Model file for the job. Use its own axes, mm. A direction names the side the tool comes from. Give positions to 0.01 mm unless a question says otherwise; leave off trailing zeros. Loops run counter-clockwise (first coordinate to the right, second up) from the corner with the lowest first, then second, coordinate; pieces in that order, holes last. Notation, with made-up numbers: M -22.75,-20.5 L 16.25,-20.5 A29 ccw 16.25,10.5 Z; hole C -24,-7.75 d8. An arc over 180 degrees is marked long. Answer in a Markdown table with one row per item.
```python
from build123d import *

# Parameters (mm, degrees)
CUT_EXTRUDE1_DEPTH = 1


with BuildPart() as part:
    # Sketch1 → Revolve1 (revolve)
    with BuildSketch(Plane(origin=(0, 0, 0), x_dir=(0, 0, -1), z_dir=(1, 0, 0)), mode=Mode.PRIVATE) as revolve1_sk:
        Polygon((0, 2.5), (0, 4.5), (-0.5, 5), (-1.5, 5), (-1.5, 4), (-12.4, 4), (-12.9, 3.5), (-12.9, 1), (-8, 1), (-8, 2.5), align=None)
    revolve(revolve1_sk.sketch.rotate(Axis((0, 0, 0), (0, 0, -1)), 90), axis=Axis((0, 0, 0), (0, 0, -1)))

    # Sketch2 → Cut-Extrude1 (cut)
    with BuildSketch(Plane(origin=(0, 4, 0), x_dir=(1, 0, 0), z_dir=(0, 1, 0))):
        with BuildLine():
            Line((-1, -12.9), (-1, -4.5))
            ThreePointArc((-1, -4.5), (0, -3.5), (1, -4.5))
            Line((1, -4.5), (1, -12.9))
            ThreePointArc((1, -12.9), (0, -13.9), (-1, -12.9))
        make_face()
    extrude(amount=-CUT_EXTRUDE1_DEPTH, mode=Mode.SUBTRACT)


solid = part.part
```
Q1. 3-axis set-ups, long thin cutter, end or side, ignore diameter. For faces 1 (the face through (-2.5, -0.1, 3.9)), 2 (the face through (2.15, -3.373, 7.026)), 3 (the face through (-1, 3.4, 8.8)), 4 (the face through (-2, 2, 0)): which of +Z, -Z, +X, -X, +Y, -Y reach the whole face in a straight line?
Reported:
| item | result |
|---|---|
| face 1 | -Z |
| face 2 | +Z |
| face 3 | +Z, +Y |
| face 4 | -Z, +X, -X, +Y, -Y |
Q2. Probe probe 1 along Y at (x, z) = (0, 2.25); probe 2 along Z at (x, y) = (1, -1.75); probe 3 along Y at (x, z) = (0, 9.15). List the from-to ranges inside material, lowest first.
Reported:
| item | result |
|---|---|
| probe 1 | -4 to -2.5, 2.5 to 4 |
| probe 2 | 8 to 12.9 |
| probe 3 | -4 to -1, 1 to 3 |
Q3. Drop flat-ended pins along their axis: pin 1 (4.5 mm diameter, centred on x = 0, y = 0, fed in from -Z); pin 2 (1.6 mm diameter, centred on x = 0.5, z = 10.5, fed in from +Y); pin 3 (1.2 mm diameter, centred on x = 0, y = 0, fed in from -Z); pin 4 (5 mm diameter, centred on y = 3, z = 3, fed in from -X). Give the stop position or say it passes through.
Reported:
| item | result |
|---|---|
| pin 1 | z = 8 |
| pin 2 | y = 3.87 |
| pin 3 | through |
| pin 4 | x = -4.9 |
Q4. Saw through at B-B (y = 0). Give the cut face in (x, z), and give its area (3 significant figures).
Reported:
| item | result |
|---|---|
| outline | M -5,0.5 L -4.5,0 L -2.5,0 L -2.5,8 L -1,8 L -1,12.9 L -3.5,12.9 L -4,12.4 L -4,1.5 L -5,1.5 Z; M 1,8 L 2.5,8 L 2.5,0 L 4.5,0 L 5,0.5 L 5,1.5 L 4,1.5 L 4,12.4 L 3.5,12.9 L 1,12.9 Z |
| area | 55.9 mm² |
Q5. Saw through at C-C (z = 7.5). Give the cut face in (x, y).
Reported:
| item | result |
|---|---|
| outline | M -1,3 L -1,3.87 A4 ccw long 1,3.87 L 1,3 Z; hole C 0,0 d5 |
Q6. Saw through at D-D (z = 9.25). Give the cut face in (x, y), and give its area (3 significant figures).
Reported:
| item | result |
|---|---|
| outline | M -1,3 L -1,3.87 A4 ccw long 1,3.87 L 1,3 Z; hole C 0,0 d2 |
| area | 45.2 mm² |
Q7. Saw through at A-A (x = 0). Give the cut face in (y, z), and give its area (3 significant figures).
Reported:
| item | result |
|---|---|
| outline | M -5,0.5 L -4.5,0 L -2.5,0 L -2.5,8 L -1,8 L -1,12.9 L -3.5,12.9 L -4,12.4 L -4,1.5 L -5,1.5 Z; M 1,8 L 2.5,8 L 2.5,0 L 4.5,0 L 5,0.5 L 5,1.5 L 4,1.5 L 4,3.5 L 3,3.5 L 3,12.9 L 1,12.9 Z |
| area | 46.6 mm² |
